Could you check a few things on this drawing? It's one solid part, dimensions in mm from its lowest x, y, z. A direction names the side the tool comes from. Coordinates: 2 decimals unless noted, no trailing zeros. Order: outer loops, then holes, each group sorted by start corner. A loop starts at its lowest first (then second) coordinate and runs counter-clockwise, first axis right, second up.
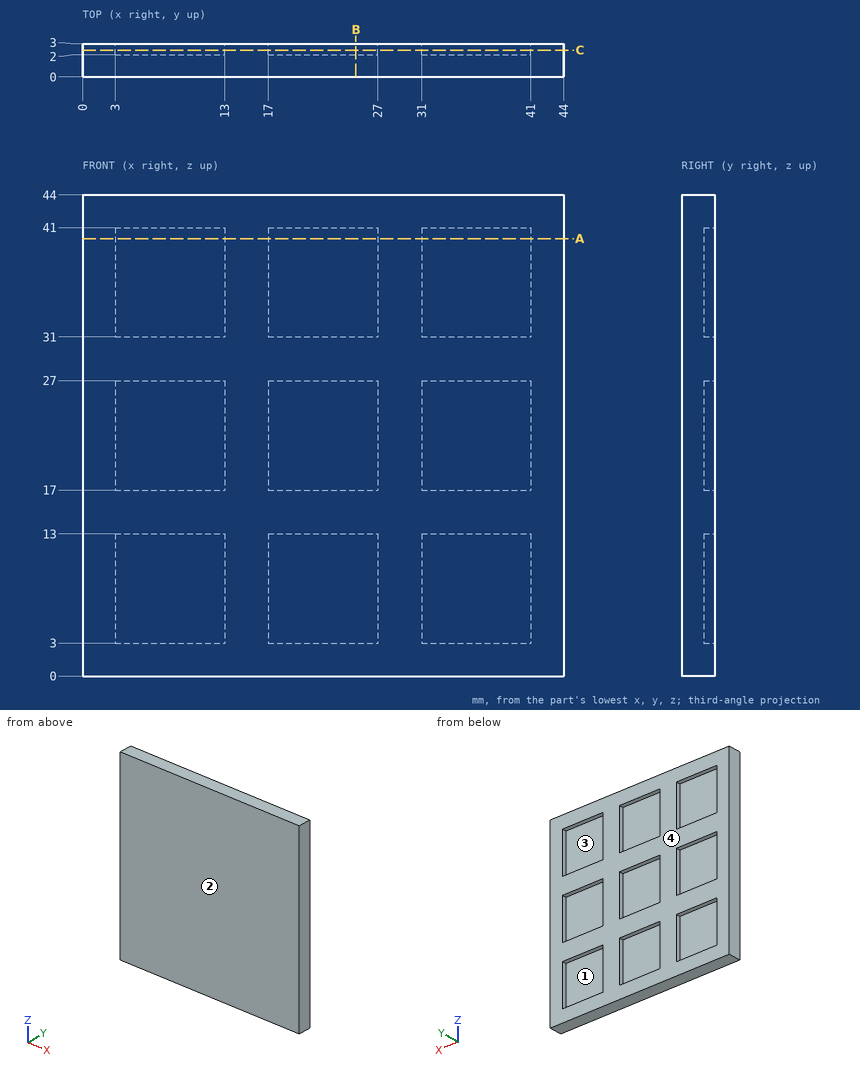
1. Please list where these lines run through material, in increasing order: probe 1 along X at (y, z) = (2.05, 24); probe 2 along Y at (x, z) = (7, 32).
Completed:
probe 1: x = 0 to 3, 13 to 17, 27 to 31, 41 to 44
probe 2: y = 0 to 2
2. Imagine slicing it at C-C on y = 2.45. Give the number of separate pieces and of enclosed holes in the cut face, then the cut area to 3 significant figures.
Completed:
separate pieces: 1
enclosed holes: 9
area: 1,040 mm2
3. On a 3-axis mill with a long thin cutter (end or side, diameter ignored), from which of +Z, -Z, +X, -X, +Y, -Y can I reach the whole of each face in a straight line? I mean the marked faces 1 and 2. Say none if no direction works.
Completed:
face 1: +Y
face 2: +Z, -Z, +X, -X, -Y
4. Thinking about a two-plate mould opening in X: for the marked faces 3 and 4, which applies, pulls with the +X half, pulls with the -X half, needs draft (parallel to the pull), parting line crosses it, or undercut?
Completed:
face 3: undercut
face 4: needs draft
5. Imagine slicing it at B-B on x = 25. Please give me the cut outline in (y, z).
Completed:
outline: (0, 0) - (3, 0) - (3, 3) - (2, 3) - (2, 13) - (3, 13) - (3, 17) - (2, 17) - (2, 27) - (3, 27) - (3, 31) - (2, 31) - (2, 41) - (3, 41) - (3, 44) - (0, 44) - close
6. I'm going to push a flat-ended pin straight in: pin 1 (3 mm diameter, centred on x = 7.5, z = 35, fed in from +Y). Where does the tip first touch, or does it pass through?
Completed:
pin 1: stops at y = 2
7. Imagine slicing it at A-A on z = 40. Please give me the cut outline in (x, y), then the cut area to 3 significant figures.
Completed:
outline: (0, 0) - (44, 0) - (44, 3) - (41, 3) - (41, 2) - (31, 2) - (31, 3) - (27, 3) - (27, 2) - (17, 2) - (17, 3) - (13, 3) - (13, 2) - (3, 2) - (3, 3) - (0, 3) - close
area: 102 mm2
